from build123d import *

# Parameters (mm, degrees)
F0_R     = 26.859981
F1_DEPTH = 81.788
F2_R     = 9.656854
F3_SIZE  = 5


with BuildPart() as f1:
    # F0 (on Top) → F1 (new body)
    with BuildSketch(Plane.XY):
        with Locations((-7.893364, 8.01296)):
            Circle(F0_R)
    extrude(amount=F1_DEPTH)

    # F2
    f2_edges = [f1.edges().sort_by_distance(p)[0] for p in [
        (-34.753345, 8.01296, 81.788),
    ]]
    fillet(f2_edges, radius=F2_R)

    # F3
    f3_edges = [f1.edges().sort_by_distance(p)[0] for p in [
        (-34.753345, 8.01296, 0),
    ]]
    chamfer(f3_edges, length=F3_SIZE)


solid = f1.part
The listing builds one solid part. Answer for the finished solid, in the listing's coordinates (mm). Coordinates: 2 decimals unless noted, no trailing zeros. Loops run counter-clockwise (first coordinate to the right, second up) from the corner with the lowest first, then second, coordinate; pieces in that order, holes last. Notation, with made-up numbers: (-31.75, -34.75) -> (0.25, -34.75) arc R27 cw to (0.25, -6.75) -> close; hole circle Ø3 at (-40, 70.5). An arc over 180 degrees is marked (long way). Answer in a Markdown table with one row per item. Add a question column.
1. Flat-ended cylindrical pins translate along their axes: P1, Ø8, axis at x = -18.5, z = 71, coming from the -Y side; P2, Ø2, axis at y = 2.5, z = 44.5, coming from the +X side. Find the tip coordinate at first contact, or state that the pin passes through.
2. Consider line 1 (Z direction, x = 7, y = -1.5); line 2 (Y direction, x = -23, z = 35.5); line 3 (Y direction, x = -14, z = 13). Determine where each line is inside the solid, lowest interval first. Write a range as [from, to].
3. The part is cut by section A-A, the plane z = 21.5. Write down the section's boundary in (x, y), then the cut area to 3 significant figures.
Answer below:
| question | item | result |
|---|---|---|
| 1 | P1 | y = -18.02 |
| 1 | P2 | x = 18.58 |
| 2 | line 1 | [0, 81.78] |
| 2 | line 2 | [-14.2, 30.22] |
| 2 | line 3 | [-18.14, 34.17] |
| 3 | outline | circle Ø53.72 at (-7.89, 8.01) |
| 3 | area | 2,270 mm2 |
